Job drawing, mm, ordinate dimensions from the low corner. One solid piece. A direction names the side the tool comes from. Round coordinates to 2 decimals unless told otherwise and drop trailing zeros. Write each loop counter-clockwise with the first axis right and the second up, starting at its lowest first coordinate (ties: lowest second). Pieces come first, ordered by that corner, then holes.
1) Which spindle directions (+Z, -Z, +X, -X, +Y, -Y) get a long thin tool onto all of the face, cutting with end or side? Do the marked faces 1, 2 and 3. Say none if no direction does.
2) Flat gauge pins, fed straight in: pin 1 (8 mm diameter, centred on x = 105, y = 26, fed in from +Z); pin 2 (12.5 mm diameter, centred on x = 39.5, z = 75, fed in from +Y); pin 3 (20 mm diameter, centred on y = 74, z = 76.5, fed in from -X). Where does each tip first touch, or does it go through?
3) Saw through at A-A on z = 73. Write the cut outline in (x, y), and give its area (3 significant figures).
4) Drill centre lines: L1, parallel to Y at x = 63.5, z = 76; L2, parallel to Y at x = 41, z = 61. Where is each one in solid material? Low to high.
5) Pull direction Y, two halves, no side cores. Call the marked faces 4, 5, 6 and 7: +Y half, -Y half, draft (parallel to the pull), parting line (faces both ways), or undercut.
6) Saw through at B-B on y = 14.5. Write the cut outline in (x, z), and give its area (3 significant figures).
7) Saw through at D-D on z = 39. Write the cut outline in (x, y).
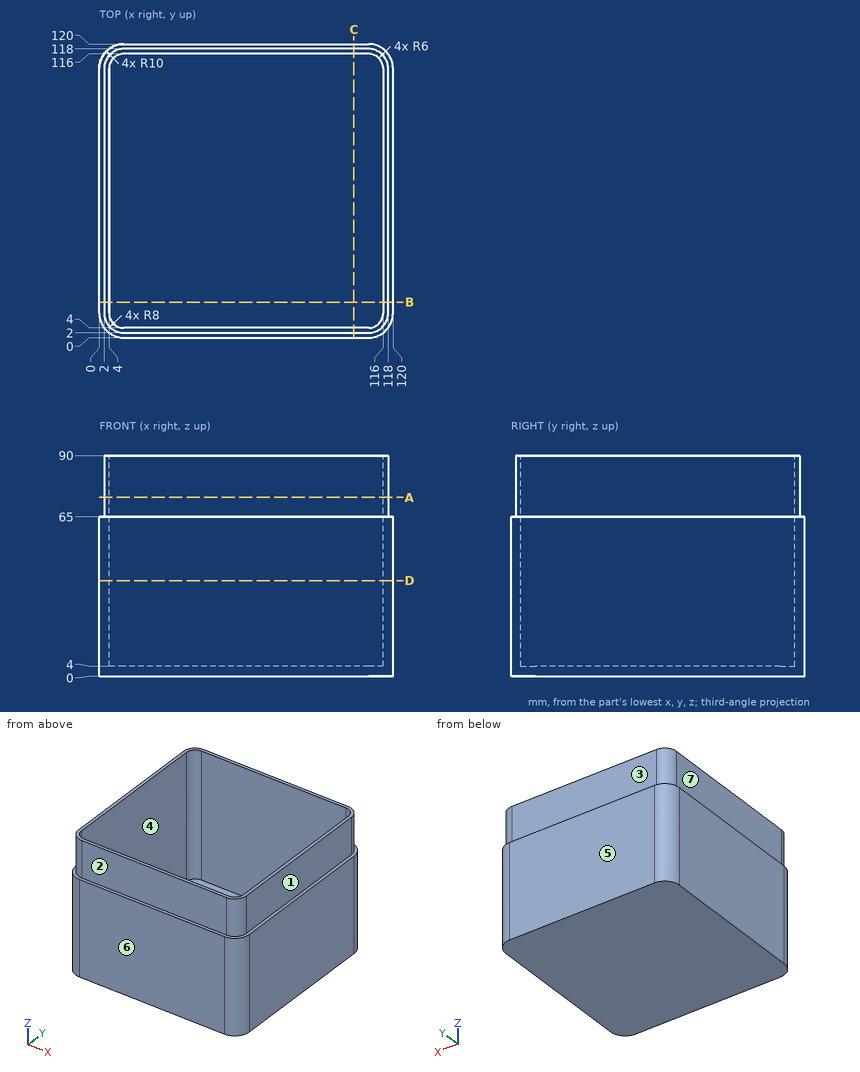
Completed:
1. face 1: +Z, +X, +Y, -Y
1. face 2: +Z, +X, -X, -Y
1. face 3: +Z, +X, -X, +Y
2. pin 1: stops at z = 4
2. pin 2: stops at y = 118
2. pin 3: stops at x = 2
3. outline: (2, 10) arc R8 ccw to (10, 2) - (110, 2) arc R8 ccw to (118, 10) - (118, 110) arc R8 ccw to (110, 118) - (10, 118) arc R8 ccw to (2, 110) - close; hole (4, 10) arc R6 ccw to (10, 4) - (110, 4) arc R6 ccw to (116, 10) - (116, 110) arc R6 ccw to (110, 116) - (10, 116) arc R6 ccw to (4, 110) - close
3. area: 888 mm2
4. L1: y = 2 to 4, 116 to 118
4. L2: y = 0 to 4, 116 to 120
5. face 4: undercut
5. face 5: +Y half
5. face 6: -Y half
5. face 7: draft
6. outline: (0, 0) - (120, 0) - (120, 65) - (118, 65) - (118, 90) - (116, 90) - (116, 4) - (4, 4) - (4, 90) - (2, 90) - (2, 65) - (0, 65) - close
6. area: 1,070 mm2
7. outline: (0, 10) arc R10 ccw to (10, 0) - (110, 0) arc R10 ccw to (120, 10) - (120, 110) arc R10 ccw to (110, 120) - (10, 120) arc R10 ccw to (0, 110) - close; hole (4, 10) arc R6 ccw to (10, 4) - (110, 4) arc R6 ccw to (116, 10) - (116, 110) arc R6 ccw to (110, 116) - (10, 116) arc R6 ccw to (4, 110) - close
